```python
from build123d import *

# Parameters (mm, degrees)
SKETCH1_R      = 2.067
BASENUT_DEPTH  = 3.52
EXTRUDE1_START = 3.68
SKETCH2_R      = 3.89
SKETCH2_R_2    = 2.067
EXTRUDE1_DEPTH = 3.68
CHAMFER1_SIZE  = 0.1556


with BuildPart() as part:
    # Sketch1 → BaseNut (new body)
    with BuildSketch(Plane.XY):
        Polygon((2.309401077, -4), (4.618802154, 0), (2.309401077, 4), (-2.309401077, 4), (-4.618802154, 0), (-2.309401077, -4), align=None)
        Circle(SKETCH1_R, mode=Mode.SUBTRACT)
    extrude(amount=-BASENUT_DEPTH)

    # Sketch3 → Double-Chamfer (revolve, cut)
    with BuildSketch(Plane(origin=(0, 0, 0), x_dir=(1, 0, 0), z_dir=(0, 1, 0))):
        Polygon((4, 3.52), (4.618802154, 3.52), (4.618802154, 3.16273441), align=None)
        Polygon((4.618802154, 0.35726559), (4, 0), (4.618802154, 0), align=None)
    revolve(axis=Axis((0, 0, -16.31077227), (0, 0, 1)), mode=Mode.SUBTRACT)

    # Sketch2 → Extrude1 (add)
    with BuildSketch(Plane(origin=(19.181370739, 9.516836059, 0), x_dir=(1, 0, 0), z_dir=(0, 0, 1)).offset(EXTRUDE1_START)):
        with Locations((-19.181370739, -9.516836059)):
            Circle(SKETCH2_R)
        with Locations((-19.181370739, -9.516836059)):
            Circle(SKETCH2_R_2, mode=Mode.SUBTRACT)
    extrude(amount=-EXTRUDE1_DEPTH)

    # Sketch5 → EndChamfer (revolve, cut)
    with BuildSketch(Plane(origin=(0, 0, 0), x_dir=(1, 0, 0), z_dir=(0, 1, 0))):
        Polygon((2.067, 3.52), (2.875, 3.52), (2.067, 3.053500982), align=None)
    revolve(axis=Axis((0, 0, -16.800797033), (0, 0, 1)), mode=Mode.SUBTRACT)

    # Chamfer1
    chamfer1_edges = [part.edges().sort_by_distance(p)[0] for p in [
        (-3.89, 0, 3.68),
    ]]
    chamfer(chamfer1_edges, length=CHAMFER1_SIZE)


solid = part.part
```
Source: CAD feature listing. Evaluate the final solid. Frame: model axes, mm. Coordinates: 2 decimals unless noted, no trailing zeros. Use a Markdown table: item, result. Add a question column.
Q1. Material intervals for L1, parallel to Y at x = 0, z = 0.5; L2, parallel to X at y = 1.75, z = 3.25; L3, parallel to X at y = -1.5, z = -3, sorted ascending.
Q2. Draft query along Y for faces 1 (the conical face through (-4.148, 0.01, -0.085)), 2 (the cylindrical face through (-1.64, -1.26, 0.36)), 3 (the conical face through (2.065, -3.597, -3.435)). Return one class per face: pulls with the +Y half, pulls with the -Y half, needs draft (parallel to the pull), parting line crosses it, or undercut.
Q3. First-contact query: pin 1 (3 mm diameter, centred on y = -3, z = 0, fed in from -X); pin 2 (4 mm diameter, centred on y = -3, z = -1, fed in from +X). Flat tips, straight axial feed; report the tip coordinate or a pass-through.
Result:
| question | item | result |
|---|---|---|
| 1 | L1 | y = -3.89 to -2.07, 2.07 to 3.89 |
| 1 | L2 | x = -3.47 to -1.1, 1.1 to 3.47 |
| 1 | L3 | x = -3.75 to -1.42, 1.42 to 3.75 |
| 2 | face 1 | parting line crosses it |
| 2 | face 2 | undercut |
| 2 | face 3 | pulls with the -Y half |
| 3 | pin 1 | stops at x = -3.75 |
| 3 | pin 2 | stops at x = 4.04 |
